The model under review builds one solid part; all positions refer to its coordinate system, in mm. Face numbers are marked on the shaded views. A direction names the side the tool comes from. Round coordinates to 2 decimals unless told otherwise and drop trailing zeros. Loops run counter-clockwise (first coordinate to the right, second up) from the corner with the lowest first, then second, coordinate; pieces in that order, holes last. Notation, with made-up numbers: (-23.75, 64) -> (-10.75, 64) arc R29 cw to (-10.75, 103) -> close; hole circle Ø4 at (55.5, -38.5). An arc over 180 degrees is marked (long way). Use a Markdown table: item, result. Add a question column.
1) For the marked faces 4, 5, 6 and 7, list the 3-axis set-ups (+Z, -Z, +X, -X, +Y, -Y) from which the entire face can be reached by the end or side of a thin tool; tool diameter is ignored.
2) Mouldability with a two-part tool opening along Y and no side actions: class the marked faces 1, 2 and 3 as released by +Y, released by -Y, zero draft, split by the parting line, or undercut.
3) Wall thickness on probe 1 along X at (y, z) = (5.5, 10); probe 2 along Y at (x, z) = (35.6, 6); probe 3 along Y at (x, z) = (38.75, 6): over which ranges is each line inside the solid? List them lowest first.
4) Insertion check: pin 1 (6 mm diameter, centred on y = 0, z = 7, fed in from -X); pin 2 (1.5 mm diameter, centred on x = 26.5, z = 11, fed in from -Y); pin 3 (5 mm diameter, centred on x = 32, z = 6, fed in from -Y); pin 4 (6 mm diameter, centred on y = 0, z = 4.5, fed in from +X). Each pin has a flat end and moves straight along its axis. Give the tip position at first contact, or say it passes through.
5) Consider section B-B on z = 6. State how many separate pieces and enclosed holes the cut face has, plus the area to 3 significant figures.
6) Consider section A-A on y = 21. Give the boundary of the cut face in (x, z).
Autodesk Inventor part; units mm, degrees
ref_plane "Work Plane1" through (41.563666, 32.216878, 0) normal (0.5, 0.8660254, 0) x (-0.8660254, 0.5, 0)
ref_plane "Work Plane2" through (44.063666, 27.886751, 0) normal (1, 0, 0) x (0, 1, 0)
ref_plane "YZ Plane" through (0, 0, 0) normal (1, 0, 0) x (0, 1, 0)
sketch "Sketch1" plane through (0, 0, 0) normal (0, 0, 1) x (1, 0, 0)
  line L0 (44.063666, 0) -> (0, 0)
  line L1 (0, 0) -> (34.830781, 60.328682)
  line L2 (34.063666, 0) -> (34.063666, 22.113249)
  line L3 (31.563666, 26.443376) -> (19.341234, 33.5)
  line L4 (44.063666, 0) -> (44.063666, 27.886751)
  line L5 (41.563666, 32.216878) -> (24.341234, 42.160254)
  arc A0 (34.063666, 22.113249) -> (31.563666, 26.443376) centre (29.063666, 22.113249) ccw
  arc A1 (44.063666, 27.886751) -> (41.563666, 32.216878) centre (39.063666, 27.886751) ccw
  line L6 (24.341234, 42.160254) -> (19.341234, 33.5)
  line L7 (24.341234, 42.160254) -> (41.563666, 32.216878)
  line L8 (19.341234, 33.5) -> (31.563666, 26.443376)
  line L9 (34.063666, 0) -> (44.063666, 0)
  line L10 (44.063666, 0) -> (44.063666, 27.886751)
  line L11 (34.063666, 0) -> (44.063666, 0)
  line L12 (44.063666, 0) -> (44.063666, 27.886751)
  line L13 (41.563666, 32.216878) -> (24.341234, 42.160254)
  line L14 (24.341234, 42.160254) -> (19.341234, 33.5)
  line L15 (19.341234, 33.5) -> (31.563666, 26.443376)
  line L16 (34.063666, 22.113249) -> (34.063666, 0)
  point P0 (25, 43.30127)
  point P1 (34.063666, 25)
  dimension "d37" = 60
  dimension "d38" = 10
  dimension "d39" = 10
  dimension "d40" = 0
  dimension "d41" = 0
  dimension "d42" = 25
  dimension "d43" = 17
  dimension "d44" = 120
  dimension "d45" = 5
extrude "Extrusion1" add sketch "Sketch1" along normal blind 12 contours L0 L2 A0 L3 L1 L5 A1 L4
ref_plane "Work Plane1" through (41.563666, 32.216878, 0) normal (0.5, 0.8660254, 0) x (-0.8660254, 0.5, 0)
sketch "Sketch2" plane through (41.563666, 32.216878, 0) normal (0.5, 0.8660254, 0) x (-0.8660254, 0.5, 0)
  circle A0 centre (19.886751, 6) radius 6
  line L0 (19.886751, 0) -> (19.886751, 12)
  line L1 (0, 12) -> (19.886751, 12)
  dimension "d5" = 12
  dimension "d47" = 0
  dimension "d48" = 6
extrude "Extrusion2" add sketch "Sketch2" against normal blind 10
ref_plane "Work Plane2" through (44.063666, 27.886751, 0) normal (1, 0, 0) x (0, 1, 0)
sketch "Sketch3" plane through (44.063666, 27.886751, 0) normal (1, 0, 0) x (0, 1, 0)
  circle A0 centre (-27.886751, 6) radius 6
  line L0 (-27.886751, 0) -> (-27.886751, 12)
  line L1 (-27.886751, 0) -> (0, 0)
  point P0 (43.30127, 10)
  point P1 (5.613249, 12)
  dimension "d10" = 12
  dimension "d49" = 0
  dimension "d50" = 6
extrude "Extrusion3" add sketch "Sketch3" against normal blind 10
sketch "Sketch4" plane through (36.563666, 23.556624, 0) normal (-0.5, -0.8660254, 0) x (0.8660254, -0.5, 0)
  circle A0 centre (-19.886751, 6) radius 2.5
  circle A1 centre (-19.886751, 6) radius 6
  point P0 (-19.886751, 0)
  point P1 (-19.886751, 12)
  dimension "d15" = 5
extrude "Extrusion4" cut sketch "Sketch4" along normal through all both and the other way through all contours A0
sketch "Sketch5" plane through (34.063666, 27.886751, 0) normal (-1, 0, 0) x (0, 0, 1)
  circle A0 centre (6, -27.886751) radius 2.5
  arc A1 (0, -27.886751) -> (12, -27.886751) centre (6, -27.886751) ccw
  dimension "d18" = 5
extrude "Extrusion5" cut sketch "Sketch5" along normal through all both and the other way through all
sketch "Sketch6" plane through (41.563666, 32.216878, 0) normal (0.5, 0.8660254, 0) x (0.8660254, -0.5, 0)
  circle A0 centre (-19.886751, -6) radius 3.6
  circle A1 centre (-19.886751, -6) radius 2.5
  arc A2 (-19.886751, 0) -> (-19.886751, 0) centre (-19.886751, -6) ccw
  point P0 (0, -10)
  dimension "d21" = 5
  dimension "d22" = 7.2
extrude "Extrusion6" cut sketch "Sketch6" against normal blind 3 contours A0
sketch "Sketch7" plane through (36.563666, 23.556624, 0) normal (-0.5, -0.8660254, 0) x (0.8660254, -0.5, 0)
  circle A0 centre (-19.886751, 6) radius 3.6
  circle A1 centre (-19.886751, 6) radius 2.5
  arc A2 (-17.386751, 6) -> (-17.386751, 6) centre (-19.886751, 6) ccw
  point P0 (-19.886751, 0)
  dimension "d25" = 5
  dimension "d26" = 7.2
extrude "Extrusion7" cut sketch "Sketch7" along normal mid plane 6
sketch "Sketch8" plane through (34.063666, 27.886751, 0) normal (-1, 0, 0) x (0, 0, 1)
  circle A0 centre (6, -27.886751) radius 3.6
  circle A1 centre (6, -27.886751) radius 2.5
  arc A2 (8.5, -27.886751) -> (8.5, -27.886751) centre (6, -27.886751) ccw
  point P0 (0, -27.886751)
  dimension "d29" = 7.2
  dimension "d30" = 5
extrude "Extrusion8" cut sketch "Sketch8" along normal mid plane 6
sketch "Sketch9" plane through (44.063666, 27.886751, 0) normal (1, 0, 0) x (0, 0, -1)
  circle A0 centre (-6, -27.886751) radius 3.6
  circle A1 centre (-6, -27.886751) radius 2.5
  circle A2 centre (-6, -27.886751) radius 2.5
  point P0 (0, -27.886751)
  dimension "d33" = 5
  dimension "d34" = 7.2
extrude "Extrusion9" cut sketch "Sketch9" against normal blind 3
fillet "Fillet1" radius 2 16 edges at (19.1451, 45.1603, 6) (32.9524, 37.1886, 0) (43.3938, 30.3868, 0) (44.0637, 13.9434, 0) (44.0637, -6, 6) (44.0637, 13.9434, 12) (43.3938, 30.3868, 12) (32.9524, 37.1886, 12) (33.3938, 24.6132, 12) (34.0637, 11.0566, 12) (34.0637, -6, 6) (34.0637, 11.0566, 0) (33.3938, 24.6132, 0) (25.4524, 29.9717, 0) (14.1451, 36.5, 6) (25.4524, 29.9717, 12)
equation "\"d38\" = d46"
equation "\"d39\" = d46"
equation "\"d3\" = width"
equation "\"d5\" = width"
equation "\"d48\" = 0.5 * width"
equation "\"d8\" = thickness"
equation "\"d10\" = width"
equation "\"d50\" = 0.5 * width"
equation "\"d13\" = thickness"
equation "\"thickness\" = thickness_1"
equation "\"width\" = width_1"
equation "\"d46\" = 10"
properties part number "Link2"
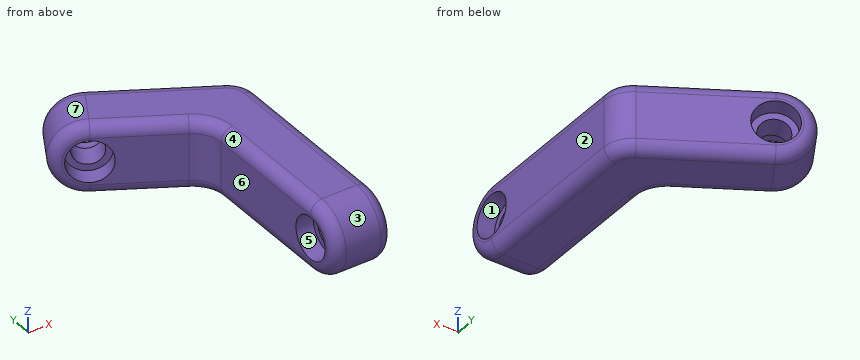
Result set:
| question | item | result |
|---|---|---|
| 1 | face 4 | +Z, -X, -Y |
| 1 | face 5 | -X |
| 1 | face 6 | +Z, -Z, -X, -Y |
| 1 | face 7 | -X, +Y |
| 2 | face 1 | undercut |
| 2 | face 2 | zero draft |
| 2 | face 3 | released by -Y |
| 3 | probe 1 | 34.06 to 44.06 |
| 3 | probe 2 | -5.95 to -3.6, 3.6 to 35.66 |
| 3 | probe 3 | -6 to -2.5, 2.5 to 33.84 |
| 4 | pin 1 | x = 34.06 |
| 4 | pin 2 | y = 29.11 |
| 4 | pin 3 | y = -5.25 |
| 4 | pin 4 | x = 44.06 |
| 5 | separate pieces | 3 |
| 5 | enclosed holes | 0 |
| 5 | area | 468 mm2 |
| 6 | outline | (34.06, 2) arc R2 ccw to (36.06, 0) -> (42.06, 0) arc R2 ccw to (44.06, 2) -> (44.06, 10) arc R2 ccw to (42.06, 12) -> (36.06, 12) arc R2 ccw to (34.06, 10) -> close |
